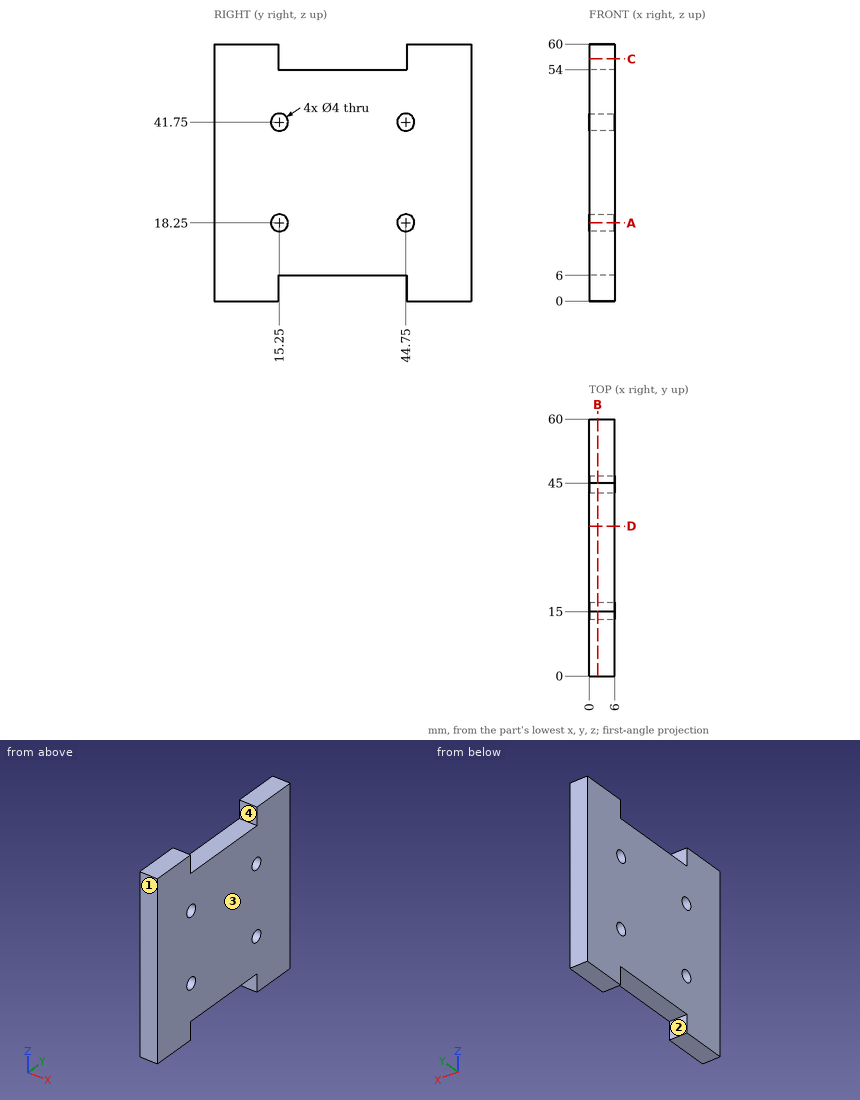
Geometry check sheet. Reference: drawing and pictorial views, mm from the part's lowest x, y, z. Give positions to 0.01 mm unless a question says otherwise; leave off trailing zeros. Order: outer loops, then holes, each group sorted by start corner. A loop starts at its lowest first (then second) coordinate and runs counter-clockwise, first axis right, second up. Notation, with made-up numbers: M 6,21 L 13,21 A16 ccw 13,28 Z; hole C 55.25,52 d7. An arc over 180 degrees is marked long. Answer as a JSON object with one key per item and string values. Group by question number.
1) Cross-section at C-C (z = 56.5). Enter the section's corners in (x, y), then the cut area to 3 significant figures.
2) Scan lines: line 1 along Y through (x, z) = (4.5, 41.75); line 2 along Y through (x, z) = (3.5, 5); line 3 along Z through (x, y) = (0.95, 14). Record each from-to range of solid material in increasing order. Write a range as [from, to].
3) Mould release check, pull along Y, two halves, no side actions. Record for the marked faces 1, 2, 3 and 4: released by +Y, released by -Y, zero draft, split by the parting line, or undercut.
4) Cross-section at A-A (z = 18.25). Enter the section's corners in (x, y).
5) Depth check by flat-ended pin: pin 1 Ø1.5 at (x, z) = (3.5, 48) entering from -Y. Enter the tip coordinate at first touch or a pass-through.
6) Cross-section at B-B (x = 2). Enter the section's corners in (y, z), then the cut area to 3 significant figures.
7) Cross-section at D-D (y = 35). Enter the section's corners in (x, z), then the cut area to 3 significant figures.
Result sheet:
{
 "1": {"outline": "M 0,0 L 6,0 L 6,15 L 0,15 Z; M 0,45 L 6,45 L 6,60 L 0,60 Z", "area": "180 mm2"},
 "2": {"line 1": "y = [0, 13.25], [17.25, 42.75], [46.75, 60]", "line 2": "y = [0, 15], [45, 60]", "line 3": "z = [0, 16.69], [19.81, 40.19], [43.31, 60]"},
 "3": {"face 1": "released by -Y", "face 2": "undercut", "face 3": "zero draft", "face 4": "undercut"},
 "4": {"outline": "M 0,0 L 6,0 L 6,13.25 L 0,13.25 Z; M 0,17.25 L 6,17.25 L 6,42.75 L 0,42.75 Z; M 0,46.75 L 6,46.75 L 6,60 L 0,60 Z"},
 "5": {"pin 1": "stops at y = 0"},
 "6": {"outline": "M 0,0 L 15,0 L 15,6 L 45,6 L 45,0 L 60,0 L 60,60 L 45,60 L 45,54 L 15,54 L 15,60 L 0,60 Z; hole C 15.25,18.25 d4; hole C 15.25,41.75 d4; hole C 44.75,18.25 d4; hole C 44.75,41.75 d4", "area": "3,190 mm2"},
 "7": {"outline": "M 0,6 L 6,6 L 6,54 L 0,54 Z", "area": "288 mm2"}
}
